Can you work these out from the model? Positions are in its coordinate system, mm. Face numbers are marked on the shaded views. Round coordinates to 2 decimals unless told otherwise and drop trailing zeros. Loops run counter-clockwise (first coordinate to the right, second up) from the corner with the lowest first, then second, coordinate; pieces in that order, holes last.
from build123d import *

# Parameters (mm, degrees)
SKETCH1_R           = 21.59
BOSS_EXTRUDE1_DEPTH = 0.79375
SKETCH2_R           = 1.4224
CUT_EXTRUDE1_DEPTH  = 31.574112518
CUT_EXTRUDE2_DEPTH  = 31.574112518


with BuildPart() as part:
    # Sketch1 → Boss-Extrude1 (new, symmetric)
    with BuildSketch(Plane(origin=(0, 0, 0), x_dir=(1, 0, 0), z_dir=(0, 1, 0))):
        with Locations(Location((0, 0, 0), (0, 0, 270))):
            Circle(SKETCH1_R)
        with BuildLine():
            Line((-3.302, 14.8779836), (-3.302, 15.5956))
            Line((-3.302, 15.5956), (3.302, 15.5956))
            Line((3.302, 15.5956), (3.302, 14.8779836))
            ThreePointArc((3.302, 14.8779836), (11.8865487, 9.537691545), (15.24, 0))
            ThreePointArc((15.24, 0), (-9.537691545, -11.8865487), (-3.302, 14.8779836))
        make_face(mode=Mode.SUBTRACT)
    extrude(amount=BOSS_EXTRUDE1_DEPTH, both=True)

    # Sketch2 → Cut-Extrude1 (cut, through all)
    with BuildSketch(Plane(origin=(0, 0.79375, 0), x_dir=(1, 0, 0), z_dir=(0, 1, 0))):
        with Locations(Location((0, 18.415, 0), (0, 0, 270))):
            Circle(SKETCH2_R)
        with Locations(Location((0, -18.415, 0), (0, 0, 270))):
            Circle(SKETCH2_R)
    extrude(amount=-CUT_EXTRUDE1_DEPTH, mode=Mode.SUBTRACT)

    # Sketch3 → Cut-Extrude2 (cut, through all)
    with BuildSketch(Plane(origin=(0, 0.79375, 0), x_dir=(1, 0, 0), z_dir=(0, 1, 0))):
        with BuildLine():
            Line((-20.871224203, 5.5245), (-16.984058744, 5.5245))
            Line((-16.984058744, 5.5245), (-16.984058744, -5.5245))
            Line((-16.984058744, -5.5245), (-20.871224203, -5.5245))
            ThreePointArc((-20.871224203, -5.5245), (-21.59, 0), (-20.871224203, 5.5245))
        make_face()
    extrude(amount=-CUT_EXTRUDE2_DEPTH, mode=Mode.SUBTRACT)


solid = part.part
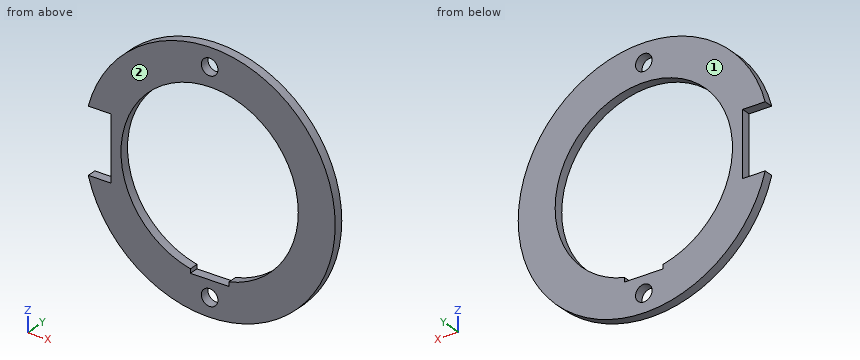
(1) If we section it at A-A, the plane z = 0: List the corners of the cut face in (x, y) for me.
Worked answers:
outline: (-16.98, -0.79) - (-15.24, -0.79) - (-15.24, 0.79) - (-16.98, 0.79) - close; (15.24, -0.79) - (21.59, -0.79) - (21.59, 0.79) - (15.24, 0.79) - close
(2) If we section it at B-B, the plane x = 0: List the corners of the cut face in (y, z) for me.
Worked answers:
outline: (-0.79, -21.59) - (0.79, -21.59) - (0.79, -19.84) - (-0.79, -19.84) - close; (-0.79, -16.99) - (0.79, -16.99) - (0.79, -15.6) - (-0.79, -15.6) - close; (-0.79, 15.24) - (0.79, 15.24) - (0.79, 16.99) - (-0.79, 16.99) - close; (-0.79, 19.84) - (0.79, 19.84) - (0.79, 21.59) - (-0.79, 21.59) - close
(3) Will these pins go through, and if not, where does the flat tip stop? P1, Ø0.5, axis at y = 0.5, z = -1.5, coming from the -X side; P2, Ø0.5, axis at x = -20, y = 0, coming from the +Z side; P3, Ø0.8, axis at y = 0, z = -15, coming from the -X side (3 decimals).
Worked answers:
P1: stops at x = -16.98
P2: stops at z = 8.72
P3: stops at x = -15.905
(4) If we section it at C-C, the plane y = -0.5: List the corners of the cut face in (x, z) for me (1 decimal), then the cut area to 3 significant figures.
Worked answers:
outline: (-20.9, -5.5) arc R21.6 ccw (long way) to (-20.9, 5.5) - (-17, 5.5) - (-17, -5.5) - close; hole (-3.3, -15.6) - (3.3, -15.6) - (3.3, -14.9) arc R15.2 ccw (long way) to (-3.3, -14.9) - close; hole circle Ø2.8 at (0, -18.4); hole circle Ø2.8 at (0, 18.4)
area: 671 mm2
(5) If we section it at D-D, the plane x = -13: List the corners of the cut face in (y, z) for me.
Worked answers:
outline: (-0.79, -17.24) - (0.79, -17.24) - (0.79, -7.95) - (-0.79, -7.95) - close; (-0.79, 7.95) - (0.79, 7.95) - (0.79, 17.24) - (-0.79, 17.24) - close
(6) If we mould it in two halves opening along Y, with no side actions, what happens to the marked faces 1 and 2? For each: released by +Y, released by -Y, zero draft, split by the parting line, or undercut.
Worked answers:
face 1: released by +Y
face 2: released by -Y
(7) If I drill on line 1 (X direction, y = -0.6, z = 19); line 2 (X direction, y = 0.3, z = 9.5); line 3 (Z direction, x = 7, y = -0.65), over which ranges is the centre line in solid material (lowest first)?
Worked answers:
line 1: x = -10.25 to -1.3, 1.3 to 10.25
line 2: x = -19.39 to -11.92, 11.92 to 19.39
line 3: z = -20.42 to -13.54, 13.54 to 20.42
